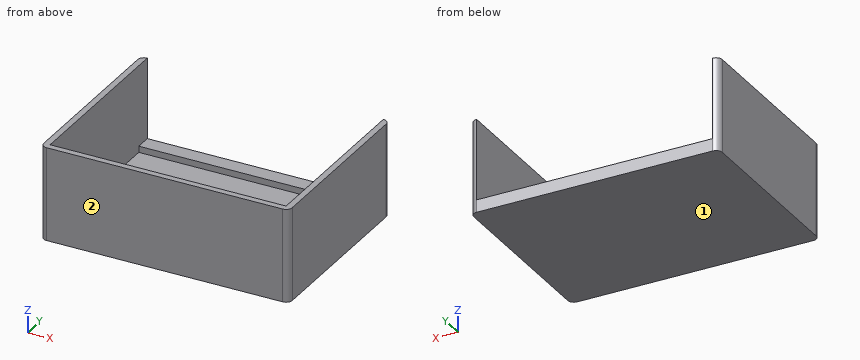
```python
from build123d import *

# Parameters (mm, degrees)
F0_W     = 400
F0_H     = 300
F1_DEPTH = 75
F2_T     = -10
F3_R     = 10
F4_R     = 10
F5_DEPTH = 25.4
F6_W     = 380
F6_H     = 25.4
F7_DEPTH = 10


with BuildPart() as f1:
    # F0 (on Top) → F1 (new body, symmetric)
    with BuildSketch(Plane.XY):
        Rectangle(F0_W, F0_H)
    extrude(amount=F1_DEPTH, both=True)

    # F2
    f2_openings = [f1.faces().sort_by_distance(p)[0] for p in [
        (0, 0, 75),
    ]]
    offset(amount=F2_T, openings=f2_openings)

    # F3
    f3_edges = [f1.edges().sort_by_distance(p)[0] for p in [
        (-200, 150, 0),
        (200, 150, 0),
    ]]
    fillet(f3_edges, radius=F3_R)

    # F4
    f4_edges = [f1.edges().sort_by_distance(p)[0] for p in [
        (200, -150, 0),
        (-200, -150, 0),
    ]]
    fillet(f4_edges, radius=F4_R)

    # F5 (cut): a face of the model
    f5_faces = [f1.faces().sort_by_distance(p)[0] for p in [
        (0, 150, 0),
    ]]
    extrude(f5_faces, amount=-F5_DEPTH, mode=Mode.SUBTRACT)

    # F6 (on face) → F7 (join, symmetric)
    with BuildSketch(Plane.XY.offset(-65)):
        with Locations((0, 137.3)):
            Rectangle(F6_W, F6_H)
    extrude(amount=F7_DEPTH, both=True)


solid = f1.part
```
Design review of the part built by this model. Coordinates are the model's own, in mm. Face numbers are marked on the shaded views. Round coordinates to 2 decimals unless told otherwise and drop trailing zeros. Order: outer loops, then holes, each group sorted by start corner. A loop starts at its lowest first (then second) coordinate and runs counter-clockwise, first axis right, second up. Notation, with made-up numbers: (50, 80) - (54, 80) arc R26 cw to (54, 116) - close; hole circle Ø10 at (-35.5, 30.25). An arc over 180 degrees is marked (long way). One line per question, with ' | ' between items.
Item 1: Wall thickness on line 1 (X direction, y = 129, z = -52); line 2 (Y direction, x = 17.5, z = -55.5); line 3 (Y direction, x = -57, z = -8.5): over which ranges is each line inside the solid? List them lowest first. Write a range as [from, to].
Checks:
line 1: [-200, -190], [190, 200] | line 2: [-150, -140], [124.6, 150] | line 3: [-150, -140]
Item 2: Take a section at B-B, the plane y = 115. Write out the cut boundary in (x, z), then the cut area to 3 significant figures.
Checks:
outline: (-200, -75) - (200, -75) - (200, 75) - (190, 75) - (190, -65) - (-190, -65) - (-190, 75) - (-200, 75) - close | area: 6,800 mm²
Item 3: Take a section at A-A, the plane x = 60. Write out the cut boundary in (y, z).
Checks:
outline: (-150, -75) - (150, -75) - (150, -55) - (124.6, -55) - (124.6, -65) - (-140, -65) - (-140, 75) - (-150, 75) - close
Item 4: For P1, Ø8, axis at x = 30.5, y = 4, coming from the +Z side; P2, Ø8, axis at x = -59.5, z = 23, coming from the +Y side; P3, Ø20.5, axis at x = -66.5, y = 133, coming from the +Z side, all flat-tipped, find the tip position at first contact; note any pin that passes through.
Checks:
P1: z = -65 | P2: y = -140 | P3: z = -55
Item 5: Draft analysis for pull direction Y (two halves, no side actions). For the marked faces 1 and 2, state which applies: +Y half, -Y half, draft (parallel to the pull), parting line (faces both ways), or undercut.
Checks:
face 1: draft | face 2: -Y half
Item 6: Take a section at C-C, the plane z = -33. Write out the cut boundary in (x, y), then the cut area to 3 significant figures.
Checks:
outline: (-200, -140) arc R10 ccw to (-190, -150) - (190, -150) arc R10 ccw to (200, -140) - (200, 140) arc R10 ccw to (190, 150) - (190, -140) - (-190, -140) - (-190, 150) arc R10 ccw to (-200, 140) - close | area: 9,710 mm²
